Part model, mm, in its own coordinate system. Face numbers are marked on the shaded views. A direction names the side the tool comes from. Give positions to 0.01 mm unless a question says otherwise; leave off trailing zeros. Write each loop counter-clockwise with the first axis right and the second up, starting at its lowest first coordinate (ties: lowest second). Pieces come first, ordered by that corner, then holes. Notation, with made-up numbers: M 87.25,20.25 L 106.25,20.25 A22 cw 106.25,53.25 Z; hole C -9,26 d7. An arc over 180 degrees is marked long. Use a Markdown table: item, result. Add a question column.
Autodesk Fusion 360 part; units mm, degrees
sketch "スケッチ1" plane through (0, 0, 0) normal (0, 1, 0) x (1, 0, 0)
  line L0 (0, -73.6187) -> (0, 8) construction
  line L1 (-8.25, -0.25) -> (-8.25, -35)
  line L2 (-8.25, -35) -> (-10.2, -35)
  line L3 (-10.2, -35) -> (-10.2, -40)
  line L4 (-10.2, -40) -> (-11.1, -40)
  line L5 (-11.1, -40) -> (-11.1, -53.75)
  line L6 (-11.35, -54) -> (-11.85, -54)
  line L7 (-12.1, -53.75) -> (-12.1, -34.3198)
  line L8 (-11.9144, -33.7395) -> (-9.4356, -30.2605)
  line L9 (-9.25, -29.6802) -> (-9.25, -0.25)
  line L10 (-9, 0) -> (-8.5, 0)
  arc A0 (-9, 0) -> (-9.25, -0.25) centre (-9, -0.25) ccw
  arc A1 (-8.25, -0.25) -> (-8.5, 0) centre (-8.5, -0.25) ccw
  arc A2 (-9.4356, -30.2605) -> (-9.25, -29.6802) centre (-10.25, -29.6802) ccw
  arc A3 (-11.9144, -33.7395) -> (-12.1, -34.3198) centre (-11.1, -34.3198) ccw
  arc A4 (-12.1, -53.75) -> (-11.85, -54) centre (-11.85, -53.75) ccw
  arc A5 (-11.35, -54) -> (-11.1, -53.75) centre (-11.35, -53.75) ccw
  point P0 (-8.25, 0)
  point P1 (-11.0999, -54)
  point P2 (-12.1, -54)
  point P3 (-12.1, -34)
  point P4 (-9.25, -30)
  point P5 (-9.25, 0)
  dimension "d5" = 5
  dimension "d6" = 14
  dimension "d7" = 35
  dimension "d8" = 1
  dimension "d9" = 1
  dimension "d10" = 20
  dimension "d11" = 30
  dimension "d12" = 0.25
  dimension "d13" = 0.25
  dimension "d16" = 1
  dimension "d17" = 1
  dimension "d18" = 0.25
  dimension "d19" = 0.25
  dimension "d23" = 8.25
  dimension "d24" = 10.2
  dimension "d25" = 11.1
revolve "回転6" add sketch "スケッチ1" angle 360 about axis through (0, 0, 73.6187) along (0, 0, -1)
revolve "回転4" [suppressed]
equation "d23 = ( 16.5 / 2 ) * 1 mm"
equation "d24 = ( 20.4 / 2 ) * 1 mm"
equation "d25 = ( 22.2 / 2 ) * 1 mm"
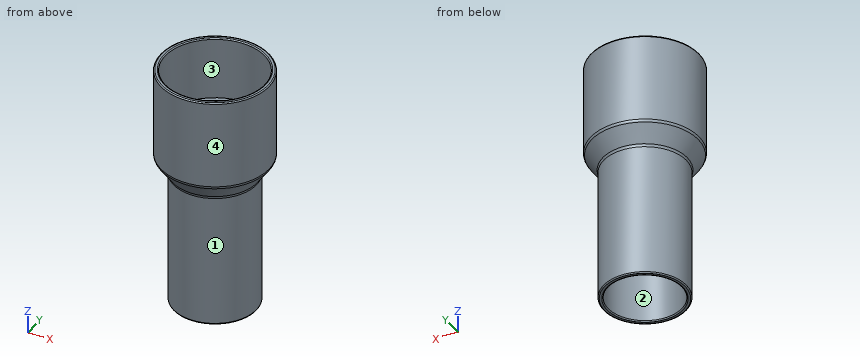
1. Mould opens along Y. For the marked faces 1 and 2 say: released by +Y, released by -Y, zero draft, split by the parting line, or undercut.
2. Cut at D-D (z = 11.5). Write the cut outline in (x, y).
3. Tool access for the marked faces 3 and 4: list every direction of +Z, -Z, +X, -X, +Y, -Y with a clear straight run to the whole face (end or side of a thin tool).
4. Cut at C-C (z = 46). Write the cut outline in (x, y), then the cut area to 3 significant figures.
5. Drill centre lines: probe 1 along Y at (x, z) = (0, 37.8); probe 2 along X at (y, z) = (0.25, 21.5); probe 3 along Y at (x, z) = (0, 44). Where is each one in solid material? Low to high. Write a range as [from, to].
6. Flat gauge pins, fed straight in: pin 1 (12 mm diameter, centred on x = 5.5, z = 28, fed in from +Y); pin 2 (3 mm diameter, centred on x = 7, z = 13, fed in from -Y); pin 3 (5 mm diameter, centred on x = 2.5, z = 27, fed in from -Y). Where does each tip first touch, or does it go through?
A:
| question | item | result |
|---|---|---|
| 1 | face 1 | split by the parting line |
| 1 | face 2 | undercut |
| 2 | outline | C 0,0 d18.5; hole C 0,0 d16.5 |
| 3 | face 3 | +Z |
| 3 | face 4 | +Z, -Z |
| 4 | outline | C 0,0 d24.2; hole C 0,0 d22.2 |
| 4 | area | 72.9 mm² |
| 5 | probe 1 | y = [-12.1, -10.2], [10.2, 12.1] |
| 5 | probe 2 | x = [-9.25, -8.25], [8.25, 9.25] |
| 5 | probe 3 | y = [-12.1, -11.1], [11.1, 12.1] |
| 6 | pin 1 | stops at y = 11.33 |
| 6 | pin 2 | stops at y = -7.44 |
| 6 | pin 3 | stops at y = -9.25 |
